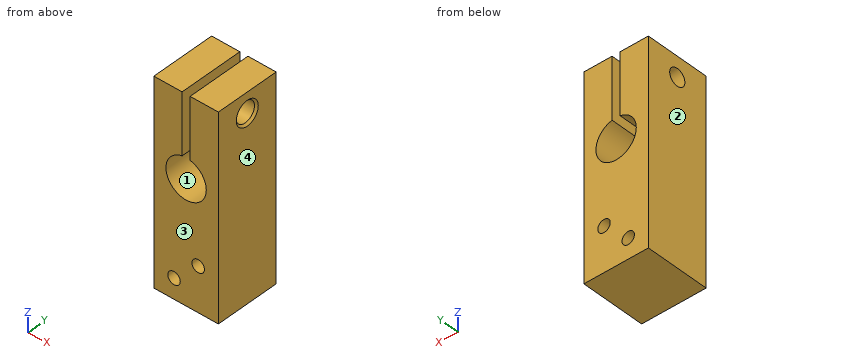
```python
from build123d import *

# Parameters (mm, degrees)
SKETCH1_W                              = 16
SKETCH1_H                              = 16
BASE_DEPTH                             = 50
SKETCH2_R                              = 5
RODSLOT_DEPTH                          = 54.103672189
RODSLOTSCREW_REACH                     = 55.104
SKETCH3_R                              = 2.55
CHAMFER1_SIZE                          = 0.5
M5X0_8_TAPPED_HOLE_FOR_ROD_SCREW_D     = 4.2
M5X0_8_TAPPED_HOLE_FOR_ROD_SCREW_DEPTH = 7.6381927
M5X0_8_TAPPED_HOLE_FOR_ROD_SCREW_TIP   = 1.2618073
SKETCH6_R                              = 1.55
SCREWSHOLES_DEPTH                      = 54.103672189


with BuildPart() as part:
    # Sketch1 → Base (new body)
    with BuildSketch(Plane.XY):
        Rectangle(SKETCH1_W, SKETCH1_H)
    extrude(amount=BASE_DEPTH)

    # Sketch2 → RodSlot (cut, through all)
    with BuildSketch(Plane(origin=(0, 8, 0), x_dir=(1, 0, 0), z_dir=(0, 1, 0))):
        with Locations((0, -30)):
            Circle(SKETCH2_R)
        with BuildLine():
            Line((-1, -34.898979486), (-1, -50))
            Line((-1, -50), (1, -50))
            Line((1, -50), (1, -34.898979486))
            ThreePointArc((1, -34.898979486), (0, -35), (-1, -34.898979486))
        make_face()
    extrude(amount=-RODSLOT_DEPTH, mode=Mode.SUBTRACT)

    # Sketch3 → RodSlotScrew (cut, up to next)
    with BuildSketch(Plane(origin=(8, 0, 0), x_dir=(0, 0, -1), z_dir=(1, 0, 0)), mode=Mode.PRIVATE) as rodslotscrew_sk1:
        with Locations((-45, 0)):
            Circle(SKETCH3_R)
    rodslotscrew_tool1 = extrude(rodslotscrew_sk1.sketch, amount=-RODSLOTSCREW_REACH, mode=Mode.PRIVATE) & part.part
    add(rodslotscrew_tool1.solids().sort_by_distance((8, 0, 45))[0], mode=Mode.SUBTRACT)

    # Chamfer1
    chamfer1_edges = [part.edges().sort_by_distance(p)[0] for p in [
        (8, 0, 47.55),
    ]]
    chamfer(chamfer1_edges, length=CHAMFER1_SIZE)

    # M5x0.8 Tapped Hole for rod screw
    with Locations(Plane.ZY.offset(8)):
        with Locations((45, 0)):
            Hole(M5X0_8_TAPPED_HOLE_FOR_ROD_SCREW_D / 2, depth=M5X0_8_TAPPED_HOLE_FOR_ROD_SCREW_DEPTH)
            with Locations((0, 0, -(M5X0_8_TAPPED_HOLE_FOR_ROD_SCREW_DEPTH + M5X0_8_TAPPED_HOLE_FOR_ROD_SCREW_TIP / 2))):  # 118° drill point
                Cone(0, M5X0_8_TAPPED_HOLE_FOR_ROD_SCREW_D / 2, M5X0_8_TAPPED_HOLE_FOR_ROD_SCREW_TIP, mode=Mode.SUBTRACT)

    # Sketch6 → ScrewsHoles (cut, through all)
    with BuildSketch(Plane.XZ.offset(8)):
        with Locations((3, 11)):
            Circle(SKETCH6_R)
        with Locations((-3, 5)):
            Circle(SKETCH6_R)
    extrude(amount=-SCREWSHOLES_DEPTH, mode=Mode.SUBTRACT)


solid = part.part
```
Source: CAD feature listing. Evaluate the final solid. Frame: model axes, mm. Face numbers are marked on the shaded views. Round coordinates to 2 decimals unless told otherwise and drop trailing zeros. Order: outer loops, then holes, each group sorted by start corner. A loop starts at its lowest first (then second) coordinate and runs counter-clockwise, first axis right, second up. Notation, with made-up numbers: (88.5, -7) -> (108.5, -7) arc R17 cw to (108.5, 16) -> close; hole circle Ø5 at (-2.5, -24.75). An arc over 180 degrees is marked (long way). One line per item, written item: value. Start each with the question number.
Q1. Section query B-B (x = -3). Return the cut outline in (y, z), plus the area to 3 significant figures.
Q2. Draft query along X for the marked faces 1, 2, 3 and 4. Return one class per face: pulls with the +X half, pulls with the -X half, needs draft (parallel to the pull), parting line crosses it, or undercut.
Q3. Pin query (flat end, axial travel): pin 1 (3 mm diameter, centred on x = -3, z = 5, fed in from +Y). Return the tip coordinate at first contact, or that it passes through.
Q4. Section query D-D (x = 7). Return the cut outline in (y, z), plus the area to 3 significant figures.
Q5. Material intervals for probe 1 along X at (y, z) = (4.75, 36); probe 2 along Z at (x, y) = (-3, -4.25); probe 3 along Z at (x, y) = (-2.5, 4), sorted ascending.
Q6. Section query A-A (y = 0). Return the cut outline in (x, z).
Q7. Section query C-C (z = 11). Return the cut outline in (x, y), plus the area to 3 significant figures.
Findings below:
1. outline: (-8, 0) -> (8, 0) -> (8, 3.45) -> (-8, 3.45) -> close; (-8, 6.55) -> (8, 6.55) -> (8, 26) -> (-8, 26) -> close; (-8, 34) -> (8, 34) -> (8, 50) -> (-8, 50) -> close; hole circle Ø4.2 at (0, 45)
1. area: 609 mm²
2. face 1: undercut
2. face 2: pulls with the -X half
2. face 3: needs draft
2. face 4: pulls with the +X half
3. pin 1: through
4. outline: (-8, 0) -> (8, 0) -> (8, 50) -> (-8, 50) -> close; hole circle Ø5.1 at (0, 45)
4. area: 780 mm²
5. probe 1: -8 to -1, 1 to 8
5. probe 2: 0 to 3.45, 6.55 to 26, 34 to 50
5. probe 3: 0 to 3.53, 6.47 to 25.67, 34.33 to 50
6. outline: (-8, 0) -> (8, 0) -> (8, 41.95) -> (7.5, 42.45) -> (1, 42.45) -> (1, 34.9) arc R5 cw (long way) to (-1, 34.9) -> (-1, 42.9) -> (-8, 42.9) -> close; (-8, 47.1) -> (-1, 47.1) -> (-1, 50) -> (-8, 50) -> close; (1, 47.55) -> (7.5, 47.55) -> (8, 48.05) -> (8, 50) -> (1, 50) -> close; hole circle Ø3.1 at (-3, 5); hole circle Ø3.1 at (3, 11)
7. outline: (-8, -8) -> (1.45, -8) -> (1.45, 8) -> (-8, 8) -> close; (4.55, -8) -> (8, -8) -> (8, 8) -> (4.55, 8) -> close
7. area: 206 mm²
